Check sheet for the modelled part. Datum: model origin and axes. Units: mm. A direction names the side the tool comes from. Give positions to 0.01 mm unless a question says otherwise; leave off trailing zeros. Write each loop counter-clockwise with the first axis right and the second up, starting at its lowest first coordinate (ties: lowest second). Pieces come first, ordered by that corner, then holes. Notation, with made-up numbers: M 23.5,48.25 L 70.5,48.25 A20 ccw 70.5,59.25 Z; hole C 52.5,-19 d6. An arc over 180 degrees is marked long. Write each question's results on one line, items separated by ' | '. Start each with the question number.
from build123d import *

# Parameters (mm, degrees)
SKETCH_2_W          = 20
SKETCH_2_H          = 25
SKETCH_2_W_2        = 1
SKETCH_2_H_2        = 1
EXTRUDE_1_DEPTH     = 3
SKETCH_3_W          = 20
SKETCH_3_H          = 3
EXTRUDE_2_DEPTH     = 10
SKETCH_5_W          = 7.5
SKETCH_5_H          = 4
SKETCH_5_W_2        = 5
CUT_EXTRUDE_1_DEPTH = 3
EXTRUDE_3_DEPTH     = 20
FILLET_1_R          = 0.2


with BuildPart() as part:
    # 草图2 → 凸台-拉伸1 (new body)
    with BuildSketch(Plane(origin=(0, 0, 0), x_dir=(1, 0, 0), z_dir=(0, 1, 0))):
        with Locations((10, 0)):
            Rectangle(SKETCH_2_W, SKETCH_2_H)
        with Locations((1.25, -7.55)):
            Rectangle(SKETCH_2_W_2, SKETCH_2_H_2, mode=Mode.SUBTRACT)
        with Locations((3.75, -7.55)):
            Rectangle(SKETCH_2_W_2, SKETCH_2_H_2, mode=Mode.SUBTRACT)
        with Locations((6.25, -7.55)):
            Rectangle(SKETCH_2_W_2, SKETCH_2_H_2, mode=Mode.SUBTRACT)
        with Locations((8.75, -7.55)):
            Rectangle(SKETCH_2_W_2, SKETCH_2_H_2, mode=Mode.SUBTRACT)
        with Locations((11.25, -7.55)):
            Rectangle(SKETCH_2_W_2, SKETCH_2_H_2, mode=Mode.SUBTRACT)
        with Locations((13.75, -7.55)):
            Rectangle(SKETCH_2_W_2, SKETCH_2_H_2, mode=Mode.SUBTRACT)
        with Locations((16.25, -7.55)):
            Rectangle(SKETCH_2_W_2, SKETCH_2_H_2, mode=Mode.SUBTRACT)
        with Locations((18.75, -7.55)):
            Rectangle(SKETCH_2_W_2, SKETCH_2_H_2, mode=Mode.SUBTRACT)
        with Locations((18.75, 7.55)):
            Rectangle(SKETCH_2_W_2, SKETCH_2_H_2, mode=Mode.SUBTRACT)
        with Locations((16.25, 7.55)):
            Rectangle(SKETCH_2_W_2, SKETCH_2_H_2, mode=Mode.SUBTRACT)
        with Locations((13.75, 7.55)):
            Rectangle(SKETCH_2_W_2, SKETCH_2_H_2, mode=Mode.SUBTRACT)
        with Locations((11.25, 7.55)):
            Rectangle(SKETCH_2_W_2, SKETCH_2_H_2, mode=Mode.SUBTRACT)
        with Locations((8.75, 7.55)):
            Rectangle(SKETCH_2_W_2, SKETCH_2_H_2, mode=Mode.SUBTRACT)
        with Locations((6.25, 7.55)):
            Rectangle(SKETCH_2_W_2, SKETCH_2_H_2, mode=Mode.SUBTRACT)
        with Locations((3.75, 7.55)):
            Rectangle(SKETCH_2_W_2, SKETCH_2_H_2, mode=Mode.SUBTRACT)
        with Locations((1.25, 7.55)):
            Rectangle(SKETCH_2_W_2, SKETCH_2_H_2, mode=Mode.SUBTRACT)
    extrude(amount=EXTRUDE_1_DEPTH)

    # 草图3 → 凸台-拉伸2 (add)
    with BuildSketch(Plane.XZ):
        with Locations((10, 11)):
            Rectangle(SKETCH_3_W, SKETCH_3_H)
        with Locations((10, -11)):
            Rectangle(SKETCH_3_W, SKETCH_3_H)
    extrude(amount=EXTRUDE_2_DEPTH)

    # 草图5 → 切除-拉伸1 (cut)
    with BuildSketch(Plane(origin=(0, 3, 0), x_dir=(1, 0, 0), z_dir=(0, 1, 0))):
        with Locations((16.25, 7.5)):
            Rectangle(SKETCH_5_W, SKETCH_5_H)
        with Locations((10, -7.5)):
            Rectangle(SKETCH_5_W_2, SKETCH_5_H)
    extrude(amount=-CUT_EXTRUDE_1_DEPTH, mode=Mode.SUBTRACT)

    # 草图4 → 凸台-拉伸3 (add)
    with BuildSketch(Plane(origin=(20, 0, 0), x_dir=(0, 0, -1), z_dir=(1, 0, 0))):
        Polygon((-12.5, -10), (-13.5, -10), (-12.5, -9), align=None)
        Polygon((9.5, -10), (8.5, -10), (9.5, -9), align=None)
        Polygon((12.5, -10), (13.5, -10), (12.5, -9), align=None)
        Polygon((-9.5, -10), (-8.5, -10), (-9.5, -9), align=None)
    extrude(amount=-EXTRUDE_3_DEPTH)

    # 圆角1
    fillet_1_edges = [part.edges().sort_by_distance(p)[0] for p in [
        (20, 3, 3.5),
        (10, 3, -12.5),
        (20, 0, 2),
        (0, -10, 11),
        (20, -10, 11),
        (0, 0, 0),
        (0, -10, -11),
        (20, 1.5, -5.5),
        (10, -10, 13.5),
        (20, -9.5, 13),
        (0, -9.5, 13),
        (0, -4.5, -9.5),
        (10, -10, -8.5),
        (0, -9.5, -9),
        (10, -10, -13.5),
        (0, -9.5, -13),
        (20, -4.5, 9.5),
        (0, -4.5, 9.5),
        (10, -10, 8.5),
        (20, -9.5, 9),
        (0, -9.5, 9),
        (0, 3, 0),
        (0, -3, -12.5),
        (20, -3, 12.5),
        (0, -3, 12.5),
        (10, 3, 12.5),
    ]]
    fillet(fillet_1_edges, radius=FILLET_1_R)


solid = part.part
Q1. Tool access check on faces 5 (the face through (0.057, -9.338, 9.248)), 6 (the face through (3.25, 1.5, 7.6)). Record the directions out of +Z, -Z, +X, -X, +Y, -Y that give a thin tool (end or side, any length) a straight path to the whole face; none if there is none.
Q2. Section check A-A on x = 3.75. Record the boundary of the cut face in (y, z), plus the area to 3 significant figures.
Q3. Section check B-B on y = -8.25. Record the boundary of the cut face in (x, z).
Q4. Release check for a two-part mould opening along Z. For faces 1 (the face through (10, 3, 0)), 2 (the face through (0.75, 1.5, 7.6)), 3 (the face through (19.943, -9.338, 12.752)), 4 (the face through (19.94, -9.335, 9.245)) record: pulls with the +Z half, pulls with the -Z half, needs draft (parallel to the pull), parting line crosses it, or undercut.
Q5. Section check D-D on x = 8.75. Record the boundary of the cut face in (y, z).
Q6. Depth check by flat-ended pin: pin 1 Ø1.1 at (x, y) = (6.5, 1) entering from +Z; pin 2 Ø0.5 at (x, y) = (13.5, 2) entering from -Z; pin 3 Ø4 at (x, z) = (16.5, -4.5) entering from -Y. Enter the tip coordinate at first touch or a pass-through.
Q7. Section check C-C on z = 5. Record the boundary of the cut face in (x, y), plus the area to 3 significant figures.
Q8. Scan lines: L1, parallel to Z at x = 13.5, y = -3.25; L2, parallel to X at y = 1, z = 6.5; L3, parallel to Y at x = 11.75, z = 2.5. Record each from-to range of solid material in increasing order.
Check result:
1) face 5: -X | face 6: +Y, -Y
2) outline: M -10,-13.02 A0.2 ccw -9.66,-13.16 L -9,-12.5 L 2.8,-12.5 A0.2 ccw 3,-12.3 L 3,-8.05 L 0,-8.05 L 0,-9.5 L -9,-9.5 L -9.66,-8.84 A0.2 ccw -10,-8.98 Z; M -10,8.98 A0.2 ccw -9.66,8.84 L -9,9.5 L 0,9.5 L 0,8.05 L 3,8.05 L 3,12.3 A0.2 ccw 2.8,12.5 L -9,12.5 L -9.66,13.16 A0.2 ccw -10,13.02 Z; M 0,-7.05 L 3,-7.05 L 3,7.05 L 0,7.05 Z | area: 131 mm^2
3) outline: M 0,-12.3 A0.2 ccw 0.2,-12.5 L 20,-12.5 L 20,-9.5 L 0.2,-9.5 A0.2 ccw 0,-9.7 Z; M 0,9.7 A0.2 ccw 0.2,9.5 L 19.8,9.5 A0.2 ccw 20,9.7 L 20,12.3 A0.2 ccw 19.8,12.5 L 0.2,12.5 A0.2 ccw 0,12.3 Z
4) face 1: needs draft | face 2: undercut | face 3: pulls with the +Z half | face 4: undercut
5) outline: M -10,-13.02 A0.2 ccw -9.66,-13.16 L -9,-12.5 L 2.8,-12.5 A0.2 ccw 3,-12.3 L 3,-8.05 L 0,-8.05 L 0,-9.5 L -9,-9.5 L -9.66,-8.84 A0.2 ccw -10,-8.98 Z; M -10,8.98 A0.2 ccw -9.66,8.84 L -9,9.5 L 3,9.5 L 3,12.3 A0.2 ccw 2.8,12.5 L -9,12.5 L -9.66,13.16 A0.2 ccw -10,13.02 Z; M 0,-7.05 L 3,-7.05 L 3,5.5 L 0,5.5 Z
6) pin 1: z = 12.5 | pin 2: z = -12.5 | pin 3: y = 0
7) outline: M 0,0.2 A0.2 ccw 0.2,0 L 19.8,0 A0.2 ccw 20,0.2 L 20,2.8 A0.2 ccw 19.8,3 L 0.2,3 A0.2 ccw 0,2.8 Z | area: 60.0 mm^2
8) L1: -12.5 to -9.5, 9.5 to 12.5 | L2: 0 to 7.5, 12.5 to 20 | L3: 0 to 3
